```python
from build123d import *

# Parameters (mm, degrees)
CROQUIS1_R                      = 45
SALIENTE_EXTRUIR1_DEPTH         = 5
CROQUIS2_R                      = 17.5
SALIENTE_EXTRUIR2_DEPTH         = 460
TALADRO_DE_MARGEN_PARA_45_D     = 3.2639
TALADRO_DE_MARGEN_PARA_45_DEPTH = 5
TALADRO_DE_MARGEN_PARA_45_TIP   = 0.980574487


with BuildPart() as part:
    # Croquis1 → Saliente-Extruir1 (new body)
    with BuildSketch(Plane(origin=(0, 0, 0), x_dir=(0, 0, -1), z_dir=(1, 0, 0))):
        Circle(CROQUIS1_R)
    extrude(amount=SALIENTE_EXTRUIR1_DEPTH)

    # Croquis2 → Saliente-Extruir2 (add)
    with BuildSketch(Plane(origin=(5, 0, 0), x_dir=(0, 0, -1), z_dir=(1, 0, 0))):
        Circle(CROQUIS2_R)
    extrude(amount=SALIENTE_EXTRUIR2_DEPTH)

    # Taladro de margen para #45
    with Locations(Plane.ZY):
        with Locations((24.168284878, 19.253675131), (-22.486191371, 20.842427824), (-23.790363973, -19.467053758), (22.632872333, -20.978386258)):
            Hole(TALADRO_DE_MARGEN_PARA_45_D / 2, depth=TALADRO_DE_MARGEN_PARA_45_DEPTH)
            with Locations((0, 0, -(TALADRO_DE_MARGEN_PARA_45_DEPTH + TALADRO_DE_MARGEN_PARA_45_TIP / 2))):  # 118° drill point
                Cone(0, TALADRO_DE_MARGEN_PARA_45_D / 2, TALADRO_DE_MARGEN_PARA_45_TIP, mode=Mode.SUBTRACT)


solid = part.part
```
Here's how the part is built. I have some questions about the finished solid (model axes, mm). A direction names the side the tool comes from. Coordinates: 2 decimals unless noted, no trailing zeros. Order: outer loops, then holes, each group sorted by start corner. A loop starts at its lowest first (then second) coordinate and runs counter-clockwise, first axis right, second up.
Item 1: I need wall thicknesses on probe 1 along X at (y, z) = (-1, -27); probe 2 along Z at (x, y) = (221.5, -0.5); probe 3 along Z at (x, y) = (49, -6). Which ranges of each line are inside material? Lowest first, please.
Response values:
probe 1: x = 0 to 5
probe 2: z = -17.49 to 17.49
probe 3: z = -16.44 to 16.44
Item 2: If we section it at D-D, the plane y = 28: List the corners of the cut face in (x, z) for me.
Response values:
outline: (0, -35.23) - (5, -35.23) - (5, 35.23) - (0, 35.23) - close
Item 3: I'm going to push flat-ended pins straight in: pin 1 Ø5 at (y, z) = (19.25, 24.17) entering from +X; pin 2 Ø12 at (x, y) = (252.5, 21.5) entering from +Z. Where does each tip first touch, or does it pass through?
Response values:
pin 1: stops at x = 5
pin 2: stops at z = 8.12
Item 4: If we section it at C-C, the plane x = 427: List the corners of the cut face in (y, z) for me.
Response values:
outline: circle Ø35 at (0, 0)
Item 5: Which directions (+Z, -Z, +X, -X, +Y, -Y) give clear straight access to the entire face, cutting with the end or side of a thin tool? Please do faces 1 (the face through (0, 1, 1)), 2 (the face through (231.78, -10.648, 13.887)).
Response values:
face 1: +Z, -Z, -X, +Y, -Y
face 2: +X
Item 6: If we section it at A-A, the plane y = 0: List the corners of the cut face in (x, z) for me.
Response values:
outline: (0, -45) - (5, -45) - (5, -17.5) - (465, -17.5) - (465, 17.5) - (5, 17.5) - (5, 45) - (0, 45) - close
